Could you check a few things on this model? Use its own coordinates, in mm. Face numbers are marked on the shaded views. A direction names the side the tool comes from. Round coordinates to 2 decimals unless told otherwise and drop trailing zeros. Loops run counter-clockwise (first coordinate to the right, second up) from the corner with the lowest first, then second, coordinate; pieces in that order, holes last. Notation, with made-up numbers: (57.25, 11.5) -> (107.25, 11.5) arc R13 ccw to (107.25, 24.5) -> close; hole circle Ø8 at (56.5, -32). An arc over 180 degrees is marked (long way). Use CSV: the item, a comma, the result in double quotes. Start each with the question number.
```python
from build123d import *

# Parameters (mm, degrees)
SKETCH10_W                = 101.6
SKETCH10_H                = 76.2
BOSS_EXTRUDE4_DEPTH       = 50.8
F_6_CLEARANCE_HOLE1_D     = 3.7973
F_6_CLEARANCE_HOLE1_DEPTH = 12.7
F_6_CLEARANCE_HOLE1_TIP   = 1.140824014
CUT_EXTRUDE6_DEPTH        = 105.726882891
BOSS_EXTRUDE6_DEPTH       = 73.025
SKETCH19_W                = 95.25
SKETCH19_H                = 69.85
CUT_EXTRUDE7_DEPTH        = 47.625
BOSS_EXTRUDE7_DEPTH       = 73.025
SKETCH21_W                = 25.4
SKETCH21_H                = 25.4
CUT_EXTRUDE8_DEPTH        = 25.4


with BuildPart() as part:
    # Sketch10 → Boss-Extrude4 (new body)
    with BuildSketch(Plane(origin=(0, 0, 0), x_dir=(1, 0, 0), z_dir=(0, 1, 0))):
        Rectangle(SKETCH10_W, SKETCH10_H)
    extrude(amount=BOSS_EXTRUDE4_DEPTH)

    # #6 Clearance Hole1
    with Locations(Plane(origin=(0, 50.8, 0), x_dir=(1, 0, 0), z_dir=(0, 1, 0))):
        with Locations((44.45, 5.55625), (44.45, -5.55625)):
            Hole(F_6_CLEARANCE_HOLE1_D / 2, depth=F_6_CLEARANCE_HOLE1_DEPTH)
            with Locations((0, 0, -(F_6_CLEARANCE_HOLE1_DEPTH + F_6_CLEARANCE_HOLE1_TIP / 2))):  # 118° drill point
                Cone(0, F_6_CLEARANCE_HOLE1_D / 2, F_6_CLEARANCE_HOLE1_TIP, mode=Mode.SUBTRACT)

    # Sketch17 → Cut-Extrude6 (cut, through all)
    with BuildSketch(Plane.XY.offset(38.1)):
        Polygon((50.8, 0), (50.8, 50.8), (37.188181024, 0), align=None)
    extrude(amount=-CUT_EXTRUDE6_DEPTH, mode=Mode.SUBTRACT)

    # Sketch18 → Boss-Extrude6 (add)
    with BuildSketch(Plane.XY.offset(38.1)):
        Polygon((47.625, 50.8), (34.013181024, 0), (37.188181024, 0), (50.8, 50.8), align=None)
    extrude(amount=-BOSS_EXTRUDE6_DEPTH)

    # Sketch19 → Cut-Extrude7 (cut)
    with BuildSketch(Plane(origin=(0, 50.8, 0), x_dir=(1, 0, 0), z_dir=(0, 1, 0))):
        Rectangle(SKETCH19_W, SKETCH19_H)
    extrude(amount=-CUT_EXTRUDE7_DEPTH, mode=Mode.SUBTRACT)

    # Sketch20 → Boss-Extrude7 (add)
    with BuildSketch(Plane.XY.offset(38.1)):
        Polygon((47.625, 50.8), (34.013181024, 0), (37.188181024, 0), (50.8, 50.8), align=None)
    extrude(amount=-BOSS_EXTRUDE7_DEPTH)

    # Sketch21 → Cut-Extrude8 (cut)
    with BuildSketch(Plane.XZ):
        with Locations((-38.1, 0)):
            Rectangle(SKETCH21_W, SKETCH21_H)
    extrude(amount=-CUT_EXTRUDE8_DEPTH, mode=Mode.SUBTRACT)


solid = part.part
```
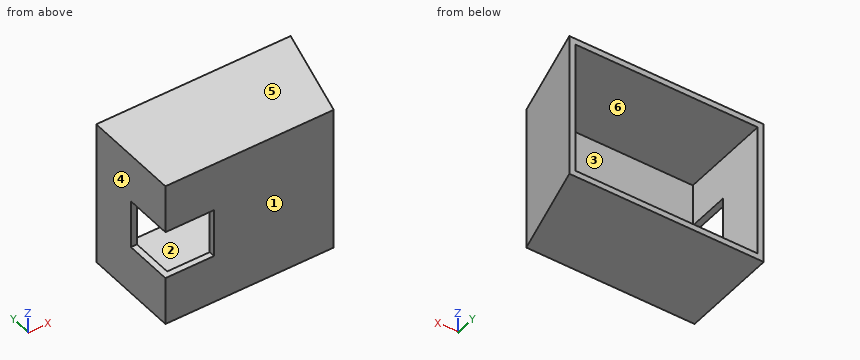
1. We'd pull the mould along X, two halves only. Please class the marked faces 3, 4, 5 and 6: pulls with the +X half, pulls with the -X half, needs draft (parallel to the pull), parting line crosses it, or undercut.
2. Suppose I cut it at B-B (x = -26.5). List the corners of the cut face in (y, z) for me (3 decimals), then the cut area to 3 significant figures.
3. If I drill on L1, parallel to Z at x = -15.5, y = 48 (3 decimals); L2, parallel to Y at x = -7, z = -22 (3 decimals); L3, parallel to X at y = 38.5, z = 10 (3 decimals), over which ranges is the centre line in solid material (lowest first)?
4. For the marked faces 1 and 2, which set-ups out of +Z, -Z, +X, -X, +Y, -Y let a thin tool reach every point of the face, with its end or its side?
5. Will these pins go through, and if not, where does the flat tip stop? pin 1 (24 mm diameter, centred on y = 28.5, z = 8, fed in from +X); pin 2 (3.5 mm diameter, centred on x = -48.5, z = -1, fed in from -Y); pin 3 (6 mm diameter, centred on x = 9, z = -24, fed in from +Y) (3 decimals).
6. Suppose I cut it at D-D (z = 20.5). List the corners of the cut face in (x, y) for me (3 decimals), then the cut area to 3 significant figures.
7. Suppose I cut it at C-C (y = 46). List the corners of the cut face in (x, z) for me (3 decimals).
8. Suppose I cut it at A-A (z = 6). List the corners of the cut face in (x, y) for me (3 decimals).
Geometry check:
1,face 3,"undercut"
1,face 4,"pulls with the -X half"
1,face 5,"needs draft"
1,face 6,"undercut"
2,outline,"(0, -38.1) -> (50.8, -38.1) -> (50.8, -34.925) -> (3.175, -34.925) -> (3.175, -12.7) -> (0, -12.7) -> close; (0, 12.7) -> (3.175, 12.7) -> (3.175, 34.925) -> (50.8, 34.925) -> (50.8, 38.1) -> (0, 38.1) -> close"
2,area,"464 mm²"
3,L1,"z = -38.1 to -34.925, 34.925 to 38.1"
3,L2,"y = 0 to 3.175"
3,L3,"x = -50.8 to -47.625, 44.329 to 47.504"
4,face 1,"+Z, -Z, +X, -X, -Y"
4,face 2,"+Y"
5,pin 1,"stops at x = 48.04"
5,pin 2,"stops at y = 25.4"
5,pin 3,"stops at y = 3.175"
6,outline,"(-50.8, 0) -> (37.188, 0) -> (50.8, 50.8) -> (47.625, 50.8) -> (34.864, 3.175) -> (-47.625, 3.175) -> (-47.625, 50.8) -> (-50.8, 50.8) -> close"
6,area,"583 mm²"
7,outline,"(-50.8, -38.1) -> (49.514, -38.1) -> (49.514, 38.1) -> (-50.8, 38.1) -> close; hole (-47.625, -34.925) -> (46.339, -34.925) -> (46.339, 34.925) -> (-47.625, 34.925) -> close"
8,outline,"(-50.8, 25.4) -> (-47.625, 25.4) -> (-47.625, 50.8) -> (-50.8, 50.8) -> close; (-25.4, 0) -> (37.188, 0) -> (50.8, 50.8) -> (47.625, 50.8) -> (34.864, 3.175) -> (-25.4, 3.175) -> close"
